```python
from build123d import *

# Parameters (mm, degrees)
F0_W     = 105
F0_H     = 60
F0_R     = 7.5
F0_R_2   = 7.5057
F1_DEPTH = 20
F2_R     = 2.5


with BuildPart() as f1:
    # F0 (on Front) → F1 (new body)
    with BuildSketch(Plane.XZ):
        Rectangle(F0_W, F0_H)
        with Locations((-17.5, 0)):
            Circle(F0_R, mode=Mode.SUBTRACT)
        Circle(F0_R, mode=Mode.SUBTRACT)
        with Locations((17.5, 0)):
            Circle(F0_R_2, mode=Mode.SUBTRACT)
    extrude(amount=F1_DEPTH)

    # F2
    f2_edges = [f1.edges().sort_by_distance(p)[0] for p in [
        (-52.5, -20, 0),
        (0, -20, 30),
        (0, -20, -30),
        (52.5, -20, 0),
    ]]
    fillet(f2_edges, radius=F2_R)


solid = f1.part
```
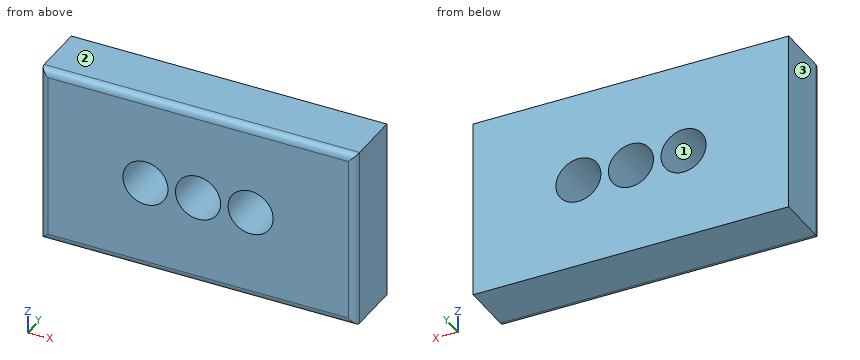
The listing builds one solid part. Answer for the finished solid, in the listing's coordinates (mm). Face numbers are marked on the shaded views. Round coordinates to 2 decimals unless told otherwise and drop trailing zeros. Loops run counter-clockwise (first coordinate to the right, second up) from the corner with the lowest first, then second, coordinate; pieces in that order, holes last. Notation, with made-up numbers: (-13.5, -28.75) - (13.5, -28.75) arc R14 ccw to (13.5, -10.75) - close; hole circle Ø3 at (-27, 75). An arc over 180 degrees is marked (long way). Return JSON: item names as keys, results as strings. Group by question number.
1. The part is cut by section A-A on x = 17.5. Determine the outline of the cut face in (y, z).
2. The part is cut by section C-C on y = -10.5. Determine the outline of the cut face in (x, z).
3. The part is cut by section D-D on x = -17.5. Determine the outline of the cut face in (y, z).
4. Consider probe 1 along Z at (x, y) = (17.5, -11); probe 2 along X at (y, z) = (-16.75, -6); probe 3 along X at (y, z) = (-17.75, 25.5). Determine where each line is inside the solid, lowest interval first.
5. This flat-tipped pin is pushed along its axis until it touches: P1, Ø13.5, axis at x = 0, z = 0, coming from the +Y side. Where does it stop, or does it pass through?
6. The mould has two halves that part along X. Classify the marked faces 1, 2 and 3: pulls with the +X half, pulls with the -X half, needs draft (parallel to the pull), parting line crosses it, or undercut.
7. The part is cut by section B-B on z = 0. Determine the outline of the cut face in (x, y), then the cut area to 3 significant figures.
Resolved:
{
 "1": {"outline": "(-20, -27.5) arc R2.5 ccw to (-17.5, -30) - (0, -30) - (0, -7.51) - (-20, -7.51) - close; (-20, 7.51) - (0, 7.51) - (0, 30) - (-17.5, 30) arc R2.5 ccw to (-20, 27.5) - close"},
 "2": {"outline": "(-52.5, -30) - (52.5, -30) - (52.5, 30) - (-52.5, 30) - close; hole circle Ø15 at (-17.5, 0); hole circle Ø15 at (0, 0); hole circle Ø15.01 at (17.5, 0)"},
 "3": {"outline": "(-20, -27.5) arc R2.5 ccw to (-17.5, -30) - (0, -30) - (0, -7.5) - (-20, -7.5) - close; (-20, 7.5) - (0, 7.5) - (0, 30) - (-17.5, 30) arc R2.5 ccw to (-20, 27.5) - close"},
 "4": {"probe 1": "z = -30 to -7.51, 7.51 to 30", "probe 2": "x = -52.5 to -22, -13 to -4.5, 4.5 to 12.99, 22.01 to 52.5", "probe 3": "x = -52.49 to 52.49"},
 "5": {"P1": "passes through"},
 "6": {"face 1": "undercut", "face 2": "needs draft", "face 3": "pulls with the -X half"},
 "7": {"outline": "(-52.5, -17.5) arc R2.5 ccw to (-50, -20) - (-25, -20) - (-25, 0) - (-52.5, 0) - close; (-10, -20) - (-7.5, -20) - (-7.5, 0) - (-10, 0) - close; (7.5, -20) - (9.99, -20) - (9.99, 0) - (7.5, 0) - close; (25.01, -20) - (50, -20) arc R2.5 ccw to (52.5, -17.5) - (52.5, 0) - (25.01, 0) - close", "area": "1,200 mm²"}
}
